Verification items for the finished model (mm, model axes). Face numbers are marked on the shaded views. A direction names the side the tool comes from. Round coordinates to 2 decimals unless told otherwise and drop trailing zeros. Order: outer loops, then holes, each group sorted by start corner. A loop starts at its lowest first (then second) coordinate and runs counter-clockwise, first axis right, second up. Notation, with made-up numbers: (14.5, -9.5) -> (47.5, -9.5) arc R35 ccw to (47.5, 26.5) -> close; hole circle Ø11 at (-5, 29.25). An arc over 180 degrees is marked (long way). Put each result on its own line as item: value.
```python
from build123d import *

# Parameters (mm, degrees)
CUT_EXTRUDE1_DEPTH      = 51
CUT_EXTRUDE2_DEPTH      = 58.445626587
CUT_EXTRUDE2_DEPTH_BACK = 58.445626587
SCALE_1_SCALE           = 0.6


with BuildPart() as part:
    # Sketch1 → Revolve1 (revolve)
    with BuildSketch(Plane(origin=(0, 0, 0), x_dir=(0, 0, -1), z_dir=(1, 0, 0)), mode=Mode.PRIVATE) as revolve1_sk:
        with BuildLine():
            Line((-20, -10), (-20, -20))
            Line((-20, -20), (0, -20))
            Line((0, -20), (0, 0))
            Line((0, 0), (0, 50))
            Line((0, 50), (-20, 50))
            Line((-20, 50), (-20, 8))
            ThreePointArc((-20, 8), (-17.656854249, 2.343145751), (-12, 0))
            ThreePointArc((-12, 0), (-15.348827212, -5.520938231), (-20, -10))
        make_face()
    revolve(revolve1_sk.sketch.rotate(Axis((0, -20, 0), (0, 1, 0)), 180), axis=Axis((0, -20, 0), (0, 1, 0)))

    # Sketch4 → Cut-Extrude1 (cut)
    with BuildSketch(Plane(origin=(-8.550503583, 48.49231552, 0), x_dir=(0, 0, -1), z_dir=(0.17364817766692414, -0.9848077530122091, 0))):
        with BuildLine():
            add(Edge.make_bspline(
                [(1.59e-07, 28.378563944), (-15.257193416, 28.378564063), (-19.289037435, 13.887286477)],
                knots=[4.712388972, 4.712388972, 4.712388972, 6.015750233, 6.015750233, 6.015750233], degree=2, weights=[1, 0.79506558, 1]))
            Line((-19.289037435, 13.887286477), (8.678255984, 16.378563944))
            Line((8.678255984, 16.378563944), (19.498892761, 13.063772103))
            add(Edge.make_bspline(
                [(19.498892761, 13.063772103), (15.950697723, 28.378563819), (1.59e-07, 28.378563944)],
                knots=[3.365916951, 3.365916951, 3.365916951, 4.712388972, 4.712388972, 4.712388972], degree=2, weights=[1, 0.781808048, 1]))
        make_face()
    cut_extrude1 = extrude(amount=CUT_EXTRUDE1_DEPTH, mode=Mode.SUBTRACT)

    # Mirror1: Cut-Extrude1 across plane
    add(cut_extrude1.mirror(Plane(origin=(0, 0, 0), x_dir=(0, 0, 1), z_dir=(1, 0, 0))), mode=Mode.SUBTRACT)

    # Sketch5 → Cut-Extrude2 (cut, two sides: drawn at the far end of the back side and taken through both)
    with BuildSketch(Plane(origin=(0, 0, 0), x_dir=(0, 0, -1), z_dir=(1, 0, 0)).offset(-CUT_EXTRUDE2_DEPTH_BACK)):
        Polygon((-24.056341891, 5.761102159), (-10.062007697, 30), (-23.062007697, 30), (-1.700047737, 67), (5.299952263, 67), (20.243066063, 11.231540074), (36.223701355, 75.285993596), (-11.110548582, 82.293611227), (-55.649834593, 36.467288671), align=None)
    extrude(amount=CUT_EXTRUDE2_DEPTH + CUT_EXTRUDE2_DEPTH_BACK, mode=Mode.SUBTRACT)


with BuildPart() as part_1:
    # 缩放比例1: scaled about (0, 0, 0)
    add(part.part.scale(SCALE_1_SCALE))


solid = part_1.part
```
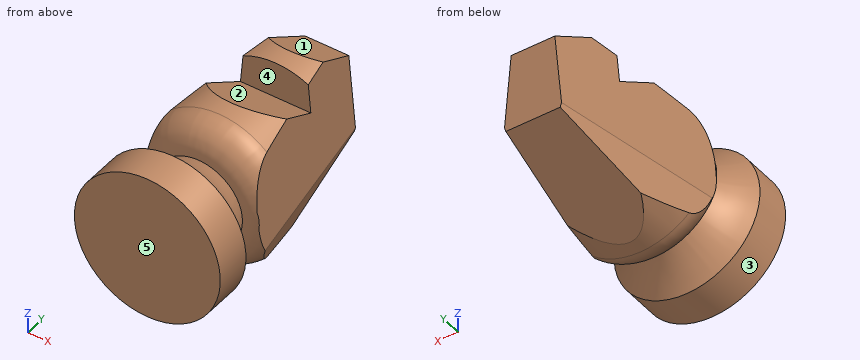
Item 1: Tool access check on the marked faces 4 and 5. Record the directions out of +Z, -Z, +X, -X, +Y, -Y that give a thin tool (end or side, any length) a straight path to the whole face; none if there is none.
Geometry check:
face 4: +Z, +X, -X
face 5: +Z, -Z, +X, -X, -Y
Item 2: Material ranges on line 1 along Y through (x, z) = (-2.75, 9.5); line 2 along Z through (x, y) = (2.5, 20.5); line 3 along X through (y, z) = (13, 6.5), recorded low to high.
Geometry check:
line 1: -12 to -4.11, 0.82 to 12, 18 to 25.51
line 2: -8.46 to 11.74
line 3: -6.63 to 6.63
Item 3: Sectioned sample at D-D, the plane y = 19. Record the boundary of the cut face in (x, z), then the cut area to 3 significant figures.
Geometry check:
outline: (-6.63, -5.21) -> (-5.49, -8.86) -> (5.49, -8.86) -> (6.63, -5.21) -> (5.18, 10.83) arc R12 ccw to (-5.18, 10.83) -> close
area: 242 mm2
Item 4: Sectioned sample at C-C, the plane z = 0. Record the boundary of the cut face in (x, y), then the cut area to 3 significant figures.
Geometry check:
outline: (-12, -12) -> (12, -12) -> (12, -6) arc R15 cw to (7.2, 0) arc R4.8 ccw to (9.54, 0.61) -> (9.4, 0.59) -> (4.22, 30) -> (-4.22, 30) -> (-9.4, 0.59) -> (-9.54, 0.61) arc R4.8 ccw to (-7.2, 0) arc R15 cw to (-12, -6) -> close
area: 665 mm2
Item 5: Sectioned sample at B-B, the plane y = 12.5. Record the boundary of the cut face in (x, z), then the cut area to 3 significant figures.
Geometry check:
outline: (-7.77, -5.21) -> (-6.2, -10.28) arc R12 ccw to (-5.62, -10.6) -> (5.62, -10.6) arc R12 ccw to (6.2, -10.28) -> (7.77, -5.21) -> (6.47, 9.21) -> (-6.47, 9.21) -> close
area: 280 mm2
Item 6: Depth check by flat-ended pin: pin 1 Ø3 at (x, y) = (8.5, 3) entering from +Z; pin 2 Ø2 at (y, z) = (13, -4.5) entering from +X; pin 3 Ø1.5 at (y, z) = (0.5, -1) entering from -X. Enter the tip coordinate at first touch or a pass-through.
Geometry check:
pin 1: z = 9.47
pin 2: x = 7.82
pin 3: x = -9.54
Item 7: Sectioned sample at A-A, the plane x = 0. Record the boundary of the cut face in (y, z), then the cut area to 3 significant figures.
Geometry check:
outline: (-12, -12) -> (-6, -12) arc R15 cw to (0, -7.2) arc R4.8 ccw to (4.8, -12) -> (7.28, -12) -> (30, -5.91) -> (30, 6.91) -> (21.18, 12) -> (18, 12) -> (18, 6.04) -> (7.67, 12) -> (4.8, 12) arc R4.8 ccw to (0, 7.2) arc R15 cw to (-6, 12) -> (-12, 12) -> close
area: 842 mm2
Item 8: Release check for a two-part mould opening along Y. For the marked faces 1, 2 and 3 record: pulls with the +Y half, pulls with the -Y half, needs draft (parallel to the pull), parting line crosses it, or undercut.
Geometry check:
face 1: pulls with the +Y half
face 2: undercut
face 3: needs draft
